Part print with two shaded views. Sizes in mm from the minimum x, y, z corner. A direction names the side the tool comes from. Round coordinates to 2 decimals unless told otherwise and drop trailing zeros. Write each loop counter-clockwise with the first axis right and the second up, starting at its lowest first coordinate (ties: lowest second). Pieces come first, ordered by that corner, then holes. Notation, with made-up numbers: (53, 64) -> (66, 64) arc R5 ccw to (66, 71) -> close; hole circle Ø3 at (-13, 68). An arc over 180 degrees is marked (long way). Return JSON: item names as keys, results as strings. Group by question number.
(1) Saw through at A-A (z = 12). List the corners of the cut face in (x, y).
(2) Mould opens along X. For the marked faces 1, 2, 3 and 4 say: +X half, -X half, draft (parallel to the pull), parting line (faces both ways), or undercut.
(3) Drill centre lines: L1, parallel to X at y = 1.8, z = 18; L2, parallel to Z at x = 45, y = 2; L3, parallel to Z at x = 60.5, y = 2.2. Where is each one in solid material? Low to high. Write a range as from..to.
(4) Saw through at C-C (y = 3.9). List the corners of the cut face in (x, z) (1 decimal).
(5) Saw through at D-D (x = 5). List the corners of the cut face in (y, z).
(6) Drop flat-ended pins along their axis: pin 1 Ø1.5 at (x, y) = (28.5, 1.5) entering from +Z; pin 2 Ø2.5 at (y, z) = (3.5, 11.5) entering from -X; pin 3 Ø1.5 at (y, z) = (1.5, 10.5) entering from +X. Give the stop position or say it passes through.
(7) Saw through at B-B (x = 30). List the corners of the cut face in (y, z), plus the area to 3 significant figures.
(8) Tool access for the marked faces 5, 6, 7 and 8: list every direction of +Z, -Z, +X, -X, +Y, -Y with a clear straight run to the whole face (end or side of a thin tool).
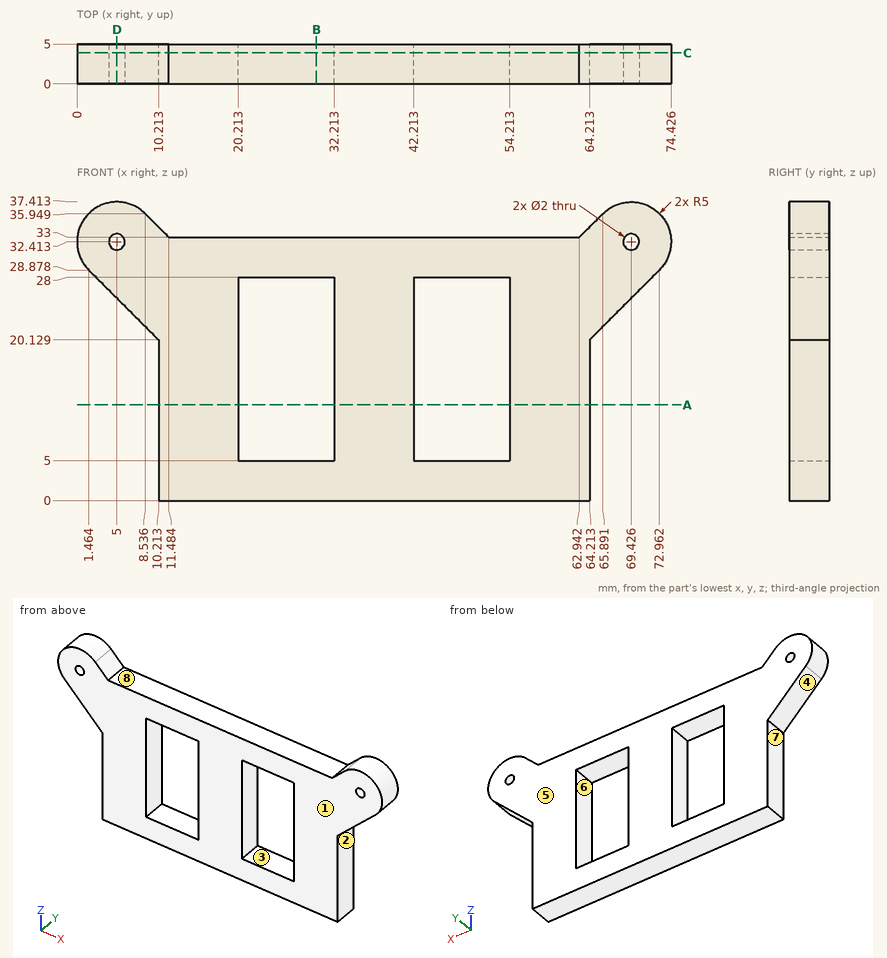
Computed values:
{
 "1": {"outline": "(10.21, 0) -> (20.21, 0) -> (20.21, 5) -> (10.21, 5) -> close; (32.21, 0) -> (42.21, 0) -> (42.21, 5) -> (32.21, 5) -> close; (54.21, 0) -> (64.21, 0) -> (64.21, 5) -> (54.21, 5) -> close"},
 "2": {"face 1": "draft", "face 2": "+X half", "face 3": "undercut", "face 4": "-X half"},
 "3": {"L1": "10.21..20.21, 32.21..42.21, 54.21..64.21", "L2": "0..5, 28..33", "L3": "0..33"},
 "4": {"outline": "(1.5, 28.9) -> (10.2, 20.1) -> (10.2, 0) -> (64.2, 0) -> (64.2, 20.1) -> (73, 28.9) arc R5 ccw to (65.9, 35.9) -> (62.9, 33) -> (11.5, 33) -> (8.5, 35.9) arc R5 ccw to start; hole circle Ø2 at (5, 32.4); hole (20.2, 5) -> (32.2, 5) -> (32.2, 28) -> (20.2, 28) -> close; hole (42.2, 5) -> (54.2, 5) -> (54.2, 28) -> (42.2, 28) -> close; hole circle Ø2 at (69.4, 32.4)"},
 "5": {"outline": "(0, 25.34) -> (5, 25.34) -> (5, 31.41) -> (0, 31.41) -> close; (0, 33.41) -> (5, 33.41) -> (5, 37.41) -> (0, 37.41) -> close"},
 "6": {"pin 1": "z = 33", "pin 2": "x = 10.21", "pin 3": "x = 64.21"},
 "7": {"outline": "(0, 0) -> (5, 0) -> (5, 5) -> (0, 5) -> close; (0, 28) -> (5, 28) -> (5, 33) -> (0, 33) -> close", "area": "50.0 mm2"},
 "8": {"face 5": "+Z, -Z, +X, -X, +Y", "face 6": "+Y, -Y", "face 7": "-Z, -X, +Y, -Y", "face 8": "+Z, +Y, -Y"}
}
